```python
from build123d import *

# Parameters (mm, degrees)
F0_R     = 36.6
F0_R_2   = 35
F0_R_3   = 14.4
F0_R_4   = 12.8
F1_DEPTH = 10
F2_R     = 36.6
F3_DEPTH = 1.6
F4_R     = 12.8
F5_DEPTH = 6
F6_W     = 40.892508
F6_H     = 6
F7_DEPTH = 8
F8_R     = 1.6
F9_DEPTH = 25


with BuildPart() as f1:
    # F0 (on Top) → F1 (new body)
    with BuildSketch(Plane.XY):
        Circle(F0_R)
        Circle(F0_R_2, mode=Mode.SUBTRACT)
        Circle(F0_R_3)
        Circle(F0_R_4, mode=Mode.SUBTRACT)
    extrude(amount=F1_DEPTH)

    # F2 (on face) → F3 (join)
    with BuildSketch(Plane.XY.offset(10)):
        Circle(F2_R)
    extrude(amount=F3_DEPTH)

    # F4 (on face) → F5 (join)
    with BuildSketch(Plane(origin=(0, 0, 10), x_dir=(1, 0, 0), z_dir=(0, 0, -1))):
        Circle(F4_R)
    extrude(amount=F5_DEPTH)

    # F6 (on face) → F7 (cut)
    with BuildSketch(Plane(origin=(0, 0, 0), x_dir=(1, 0, 0), z_dir=(0, 0, -1))):
        Rectangle(F6_W, F6_H)
    extrude(amount=-F7_DEPTH, mode=Mode.SUBTRACT)

    # F8 (on face) → F9 (cut)
    with BuildSketch(Plane(origin=(0, 0, 8), x_dir=(1, 0, 0), z_dir=(0, 0, -1))):
        Circle(F8_R)
    extrude(amount=-F9_DEPTH, mode=Mode.SUBTRACT)


solid = f1.part
```
Could you check a few things on this model? Use its own coordinates, in mm. A direction names the side the tool comes from. Coordinates: 2 decimals unless noted, no trailing zeros. Write each loop counter-clockwise with the first axis right and the second up, starting at its lowest first coordinate (ties: lowest second). Pieces come first, ordered by that corner, then holes. Notation, with made-up numbers: (-12.5, 30.25) -> (24.5, 30.25) arc R33 cw to (24.5, 58.25) -> close; hole circle Ø4 at (67, 19.5). An arc over 180 degrees is marked (long way). Return JSON: item names as keys, results as strings.
(1) Imagine slicing it at C-C, the plane y = 0. Please give me the cut outline in (x, z), then the cut area to 3 significant figures.
Numbers:
{"outline": "(-36.6, 0) -> (-35, 0) -> (-35, 10) -> (-14.4, 10) -> (-14.4, 8) -> (-1.6, 8) -> (-1.6, 11.6) -> (-36.6, 11.6) -> close; (1.6, 8) -> (14.4, 8) -> (14.4, 10) -> (35, 10) -> (35, 0) -> (36.6, 0) -> (36.6, 11.6) -> (1.6, 11.6) -> close", "area": "195 mm2"}
(2) Which directions (+Z, -Z, +X, -X, +Y, -Y) give clear straight access to the entire face, cutting with the end or side of a thin tool? Please do faces 1 (the flat face through (19, -30, 0)), 2 (the flat face through (0, -15, 10)).
Numbers:
{"face 1": "-Z, +X, -X, +Y, -Y", "face 2": "-Z"}
(3) I need wall thicknesses on L1, parallel to Y at x = 0, z = 9.7; L2, parallel to Y at x = -7.5, z = 1; L3, parallel to Z at x = 32.5, y = -9. Which ranges of each line are inside material? Lowest first, please.
Numbers:
{"L1": "y = -36.6 to -35, -14.4 to -1.6, 1.6 to 14.4, 35 to 36.6", "L2": "y = -35.82 to -34.19, -12.29 to -10.37, 10.37 to 12.29, 34.19 to 35.82", "L3": "z = 10 to 11.6"}
(4) Imagine slicing it at B-B, the plane z = 1.5. Please give me the cut outline in (x, y), then the cut area to 3 significant figures.
Numbers:
{"outline": "circle Ø73.2 at (0, 0); (-14.08, -3) arc R14.4 ccw to (14.08, -3) -> (12.44, -3) arc R12.8 cw to (-12.44, -3) -> close; (-14.08, 3) -> (-12.44, 3) arc R12.8 cw to (12.44, 3) -> (14.08, 3) arc R14.4 ccw to start; hole circle Ø70 at (0, 0)", "area": "477 mm2"}
(5) I'm going to push flat-ended pins straight in: pin 1 (8 mm diameter, centred on x = 3, y = -6.5, fed in from -Z); pin 2 (1 mm diameter, centred on x = -8, z = 10, fed in from +Y); pin 3 (4 mm diameter, centred on x = 0, z = 4.5, fed in from -Y); pin 4 (4 mm diameter, centred on x = -28.5, y = -28, fed in from +Z). Where does each tip first touch, or does it pass through?
Numbers:
{"pin 1": "stops at z = 4", "pin 2": "stops at y = 35.82", "pin 3": "stops at y = -36.6", "pin 4": "passes through"}
(6) Imagine slicing it at D-D, the plane y = 20.5. Please give me the cut outline in (x, z).
Numbers:
{"outline": "(-30.32, 0) -> (-28.37, 0) -> (-28.37, 10) -> (28.37, 10) -> (28.37, 0) -> (30.32, 0) -> (30.32, 11.6) -> (-30.32, 11.6) -> close"}
(7) Imagine slicing it at A-A, the plane x = 0. Please give me the cut outline in (y, z), then the cut area to 3 significant figures.
Numbers:
{"outline": "(-36.6, 0) -> (-35, 0) -> (-35, 10) -> (-14.4, 10) -> (-14.4, 0) -> (-12.8, 0) -> (-12.8, 4) -> (-3, 4) -> (-3, 8) -> (-1.6, 8) -> (-1.6, 11.6) -> (-36.6, 11.6) -> close; (1.6, 8) -> (3, 8) -> (3, 4) -> (12.8, 4) -> (12.8, 0) -> (14.4, 0) -> (14.4, 10) -> (35, 10) -> (35, 0) -> (36.6, 0) -> (36.6, 11.6) -> (1.6, 11.6) -> close", "area": "299 mm2"}
(8) We'd pull the mould along Y, two halves only. Please class faces 3 (the flat face through (1, 13, 0)), 4 (the flat face through (0, 7, 4)), 5 (the cylindrical face through (19.68, 30.86, 5.72)): +Y half, -Y half, draft (parallel to the pull), parting line (faces both ways), or undercut.
Numbers:
{"face 3": "draft", "face 4": "undercut", "face 5": "parting line"}
